Input: part model. Units: mm. Frame: model coordinates. A direction names the side the tool comes from. Round coordinates to 2 decimals unless told otherwise and drop trailing zeros. Loops run counter-clockwise (first coordinate to the right, second up) from the corner with the lowest first, then second, coordinate; pieces in that order, holes last. Notation, with made-up numbers: (59.25, -25) - (65.25, -25) arc R31 cw to (65.25, 3) - close; hole circle Ø4 at (-20.5, -9.75). An arc over 180 degrees is marked (long way). Use CSV: the item, a comma, the result in double quotes. Start each with the question number.
1. Cut plane B-B (x = 73). Return loops of the section in (y, z) (3 decimals), and give its area (3 significant figures).
2. Cut plane A-A (y = 14.5). Give the number of separate pieces and of enclosed holes in the cut face, and give its area (3 significant figures).
3. Access query for faces 1 (the cylindrical face through (1.49, 6.08, 30.61)), 2 (the flat face through (53, 68.494, 22)), 3 (the flat face through (106, 16, 10.858)). Directions: +Z, -Z, +X, -X, +Y, -Y. A direction counts if a zero-diameter tool reaches every point of the face in a straight line with its end or side. Return the directions, or none.
4. Material intervals for probe 1 along X at (y, z) = (42, 5.5) (3 decimals); probe 2 along X at (y, z) = (30, 6) (3 decimals); probe 3 along Y at (x, z) = (93.5, 28.5), sorted ascending. Write a range as from..to.
5. Pin query (flat end, axial travel): P1, Ø8, axis at y = 33, z = 31.5, coming from the +X side; P2, Ø4, axis at y = 48.5, z = 12.5, coming from the -X side; P3, Ø6, axis at y = 32, z = 20, coming from the +X side; P4, Ø8, axis at x = 79.5, y = 33, coming from the +Z side (3 decimals). Return the tip coordinate at first contact, or that it passes through.
```python
from build123d import *

# Parameters (mm, degrees)
F0_W      = 107.95
F0_H      = 71.5264
F1_DEPTH  = 3.175
F2_W      = 101.7524
F2_H      = 65.46088
F3_DEPTH  = 38.1
F4_W      = 17.272
F4_H      = 14.478
F4_W_2    = 9.779
F4_H_2    = 12.192
F5_DEPTH  = 3.176
F6_W      = 9.525
F6_H      = 1.5875
F7_DEPTH  = 3.175
F8_DEPTH  = 3.176
F9_W      = 2.54
F9_H      = 12.7
F10_DEPTH = 12.7
F11_R     = 1.524
F12_DEPTH = 3.0226
F13_R     = 1.143
F14_DEPTH = 41.276
F15_W     = 10.668
F15_H     = 8.255
F16_DEPTH = 3.175


with BuildPart() as f1:
    # F0 (on Top) → F1 (new body)
    with BuildSketch(Plane.XY):
        with Locations((53.975, 35.7632)):
            Rectangle(F0_W, F0_H)
    extrude(amount=F1_DEPTH)

    # F2 (on face) → F3 (join)
    with BuildSketch(Plane.XY.offset(3.175)):
        Polygon((107.95, 71.5264), (0, 71.5264), (0, 68.49364), (0, 3.03276), (0, 0), (107.95, 0), align=None)
        with Locations((53.8988, 35.7632)):
            Rectangle(F2_W, F2_H, mode=Mode.SUBTRACT)
    extrude(amount=F3_DEPTH)

    # F4 (on face) → F5 (cut, through all)
    with BuildSketch(Plane(origin=(104.775, 0, 0), x_dir=(0, -1, 0), z_dir=(-1, 0, 0))):
        with Locations((-31.5214, 16.51)):
            Rectangle(F4_W, F4_H)
        with Locations((-52.3367, 15.367)):
            Rectangle(F4_W_2, F4_H_2)
    extrude(amount=-F5_DEPTH, mode=Mode.SUBTRACT)

    # F6 (on face) → F7 (cut, through all)
    with BuildSketch(Plane.YZ.offset(107.95)):
        with Locations((15.5829, 10.06475)):
            Rectangle(F6_W, F6_H)
    extrude(amount=-F7_DEPTH, mode=Mode.SUBTRACT)

    # F4 (on face) → F8 (cut, through all)
    with BuildSketch(Plane(origin=(104.775, 0, 0), x_dir=(0, -1, 0), z_dir=(-1, 0, 0))):
        with Locations((-31.5214, 16.51)):
            Rectangle(F4_W, F4_H)
        with Locations((-52.3367, 15.367)):
            Rectangle(F4_W_2, F4_H_2)
    extrude(amount=-F8_DEPTH, mode=Mode.SUBTRACT)

    # F9 (on face) → F10 (join)
    with BuildSketch(Plane.XY.offset(3.175)):
        with Locations((16.9672, 48.17364)):
            Rectangle(F9_W, F9_H)
    extrude(amount=F10_DEPTH)

    # F11 (on face) → F12 (cut, through all)
    with BuildSketch(Plane(origin=(0, 0, 0), x_dir=(0, -1, 0), z_dir=(-1, 0, 0))):
        Polygon((-43.1673, 37.513494), (-62.9793, 37.513494), (-61.5823, 26.681205), (-44.5643, 26.681205), align=None)
        Polygon((-43.1673, 15.815138), (-62.9793, 15.815138), (-61.5823, 4.98285), (-44.5643, 4.98285), align=None)
        Polygon((-8.5471, 37.513494), (-28.3591, 37.513494), (-26.9621, 26.681205), (-9.9441, 26.681205), align=None)
        Polygon((-8.5471, 15.815138), (-28.3591, 15.815138), (-26.9621, 4.98285), (-9.9441, 4.98285), align=None)
        with Locations((-40.3733, 32.09735)):
            Circle(F11_R)
        with Locations((-65.7733, 32.09735)):
            Circle(F11_R)
        with Locations((-65.7733, 10.398994)):
            Circle(F11_R)
        with Locations((-40.3733, 10.398994)):
            Circle(F11_R)
        with Locations((-31.1531, 10.398994)):
            Circle(F11_R)
        with Locations((-5.7531, 10.398994)):
            Circle(F11_R)
        with Locations((-5.7531, 32.09735)):
            Circle(F11_R)
        with Locations((-31.1531, 32.09735)):
            Circle(F11_R)
    extrude(amount=-F12_DEPTH, mode=Mode.SUBTRACT)

    # F13 (on face) → F14 (cut, through all)
    with BuildSketch(Plane(origin=(0, 0, 0), x_dir=(1, 0, 0), z_dir=(0, 0, -1))):
        with Locations((13.335, -62.4332)):
            Circle(F13_R)
        with Locations((13.335, -35.7632)):
            Circle(F13_R)
        with Locations((13.335, -9.0932)):
            Circle(F13_R)
    extrude(amount=-F14_DEPTH, mode=Mode.SUBTRACT)

    # F15 (on face) → F16 (cut, through all)
    with BuildSketch(Plane.YZ.offset(107.95)):
        with Locations((29.4894, 27.8765)):
            Rectangle(F15_W, F15_H)
    extrude(amount=-F16_DEPTH, mode=Mode.SUBTRACT)


solid = f1.part
```
Established:
1,outline,"(0, 0) - (71.526, 0) - (71.526, 41.275) - (68.494, 41.275) - (68.494, 3.175) - (3.033, 3.175) - (3.033, 41.275) - (0, 41.275) - close"
1,area,"458 mm2"
2,separate pieces,"4"
2,enclosed holes,"0"
2,area,"508 mm2"
3,face 1,"-X"
3,face 2,"+Z"
3,face 3,"+X, -X"
4,probe 1,"x = 0..3.023, 15.697..18.237, 104.775..107.95"
4,probe 2,"x = 0..3.023, 104.775..107.95"
4,probe 3,"y = 0..3.03, 68.49..71.53"
5,P1,"stops at x = 107.95"
5,P2,"stops at x = 15.7"
5,P3,"stops at x = 3.02"
5,P4,"stops at z = 3.175"
